from build123d import *
from OCP.BRepFilletAPI import BRepFilletAPI_MakeChamfer

# Parameters (mm, degrees)
SKETCH1_R           = 2.794
SKETCH1_R_2         = 2.667
BOSS_EXTRUDE1_DEPTH = 19.05
CHAMFER1_SIZE       = 2.54
CHAMFER2_SIZE       = 2.54
CHAMFER2_SIZE2      = 1.962221924
SKETCH2_W           = 11.068186497
SKETCH2_H           = 4.064
NOTCH_DEPTH         = 11.43


with BuildPart() as part:
    # Sketch1 → Boss-Extrude1 (new body)
    with BuildSketch(Plane(origin=(0, 0, 0), x_dir=(1, 0, 0), z_dir=(0, 1, 0))):
        Polygon((-3.81, 46.459871133), (0, 46.459871133), (0, 33.759871133), (8.89, 33.759871133), (8.89, 21.59), (0, 21.59), (0, 11.43), (4.445, 0), (-8.255, 0), (-3.81, 11.43), align=None)
        with Locations(Location((2.54, 27.409871133, 0), (0, 0, 90))):
            Circle(SKETCH1_R, mode=Mode.SUBTRACT)
        with Locations(Location((-1.905, 4.445, 0), (0, 0, 90))):
            Circle(SKETCH1_R_2, mode=Mode.SUBTRACT)
    extrude(amount=BOSS_EXTRUDE1_DEPTH)

    # Chamfer1
    chamfer1_edges = [part.edges().sort_by_distance(p)[0] for p in [
        (0, 9.525, -21.59),
        (8.89, 9.525, -21.59),
        (8.89, 9.525, -33.759871133),
        (0, 9.525, -33.759871133),
    ]]
    chamfer(chamfer1_edges, length=CHAMFER1_SIZE)

    # Chamfer2: one chamfer whose edges measure the first distance from different faces: ONE call of the kernel's chamfer builder (chamfer() names one face for all edges)
    chamfer2_edges_1 = [part.edges().sort_by_distance(p)[0] for p in [
        (4.445, 9.525, 0),
    ]]
    chamfer2_side_1 = [part.faces().sort_by_distance(p)[0] for p in [
        (-1.905, 9.525, 0),
    ]]
    chamfer2_edges_2 = [part.edges().sort_by_distance(p)[0] for p in [
        (-8.255, 9.525, 0),
    ]]
    chamfer2_side_2 = [part.faces().sort_by_distance(p)[0] for p in [
        (-6.0325, 9.525, -5.715),
    ]]
    chamfer2 = BRepFilletAPI_MakeChamfer(part.part.solid().wrapped)
    for e in chamfer2_edges_1:
        chamfer2.Add(CHAMFER2_SIZE, CHAMFER2_SIZE2, e.wrapped, chamfer2_side_1[0].wrapped)  # the first distance lies on this face
    for e in chamfer2_edges_2:
        chamfer2.Add(CHAMFER2_SIZE, CHAMFER2_SIZE2, e.wrapped, chamfer2_side_2[0].wrapped)  # the first distance lies on this face
    add(Compound.cast(chamfer2.Shape()), mode=Mode.REPLACE)

    # Sketch2 → notch (cut)
    with BuildSketch(Plane.XY):
        with Locations((-1.800293249, 9.525)):
            Rectangle(SKETCH2_W, SKETCH2_H)
    extrude(amount=-NOTCH_DEPTH, mode=Mode.SUBTRACT)


solid = part.part
Verification items for the finished model (mm, model axes). A direction names the side the tool comes from. Give positions to 0.01 mm unless a question says otherwise; leave off trailing zeros. Write each loop counter-clockwise with the first axis right and the second up, starting at its lowest first coordinate (ties: lowest second). Pieces come first, ordered by that corner, then holes. Notation, with made-up numbers: M 72.5,-36.75 L 117.5,-36.75 A12 ccw 117.5,-18.75 Z; hole C 22,5.5 d11. An arc over 180 degrees is marked long. Write item = value, one per line.
(1) Sectioned sample at C-C (z = -27). Record the cut outline in (x, y).
Found:
outline = M -3.81,0 L -0.22,0 L -0.22,19.05 L -3.81,19.05 Z; M 5.3,0 L 8.89,0 L 8.89,19.05 L 5.3,19.05 Z
(2) Sectioned sample at D-D (y = 5.5). Record the cut outline in (x, z) (3 decimals), then the cut area to 3 significant figures.
Found:
outline = M -7.334,-2.367 L -3.81,-11.43 L -3.81,-46.46 L 0,-46.46 L 0,-36.3 L 2.54,-33.76 L 6.35,-33.76 L 8.89,-31.22 L 8.89,-24.13 L 6.35,-21.59 L 2.54,-21.59 L 0,-19.05 L 0,-11.43 L 3.734,-1.829 L 1.905,0 L -6.293,0 Z; hole C -1.905,-4.445 d5.334; hole C 2.54,-27.41 d5.588
area = 284 mm2
(3) Draft check along X on faces 4 (the face through (-6.806, 3.694, -1.167)), 5 (the face through (-2.706, 15.251, -6.989)), 6 (the face through (2.832, 15.251, -0.927)). Enter one of: released by +X, released by -X, zero draft, split by the parting line, or undercut.
Found:
face_4 = released by -X
face_5 = undercut
face_6 = released by +X
(4) Material ranges on line 1 (X direction, y = 4.5, z = -42.5); line 2 (Z direction, x = -2, y = 8.5); line 3 (Y direction, x = 0.25, z = -10), recorded low to high.
Found:
line_1 = -3.81 to 0
line_2 = -46.46 to -11.43
line_3 = 0 to 7.49, 11.56 to 19.05
(5) Go/stop test with flat-tipped pins: pin 1 Ø1.5 at (x, y) = (4, 16.5) entering from +Z (3 decimals); pin 2 Ø8 at (x, y) = (0.5, 15) entering from -Z; pin 3 Ø4 at (x, z) = (5, -9) entering from +Y; pin 4 Ø1.1 at (x, y) = (4, 5) entering from -Z. Record where each tip stops, or that it passes through.
Found:
pin_1 = -1.345
pin_2 = -46.46
pin_3 = through
pin_4 = -33.76
(6) Sectioned sample at A-A (x = -1). Record the cut outline in (y, z), then the cut area to 3 significant figures.
Found:
outline = M 0,-46.46 L 19.05,-46.46 L 19.05,-6.95 L 11.56,-6.95 L 11.56,-11.43 L 7.49,-11.43 L 7.49,-6.95 L 0,-6.95 Z; M 0,-1.94 L 7.49,-1.94 L 7.49,0 L 0,0 Z; M 11.56,-1.94 L 19.05,-1.94 L 19.05,0 L 11.56,0 Z
area = 763 mm2
(7) Access from +Z, -Z, +X, -X, +Y, -Y to the whole of each face (thin tool, end or side, straight path). Record for faces 1 (the face through (4, 9, -33.76)), 2 (the face through (1.25, 9.39, -20.3)), 3 (the face through (-2, 10, -11.43)).
Found:
face_1 = -Z, +X, +Y, -Y
face_2 = +X, +Y, -Y
face_3 = +Z, +X, -X
(8) Sectioned sample at B-B (x = -5.25). Record the cut outline in (y, z).
Found:
outline = M 0,-7.73 L 7.49,-7.73 L 7.49,0 L 0,0 Z; M 11.56,-7.73 L 19.05,-7.73 L 19.05,0 L 11.56,0 Z
